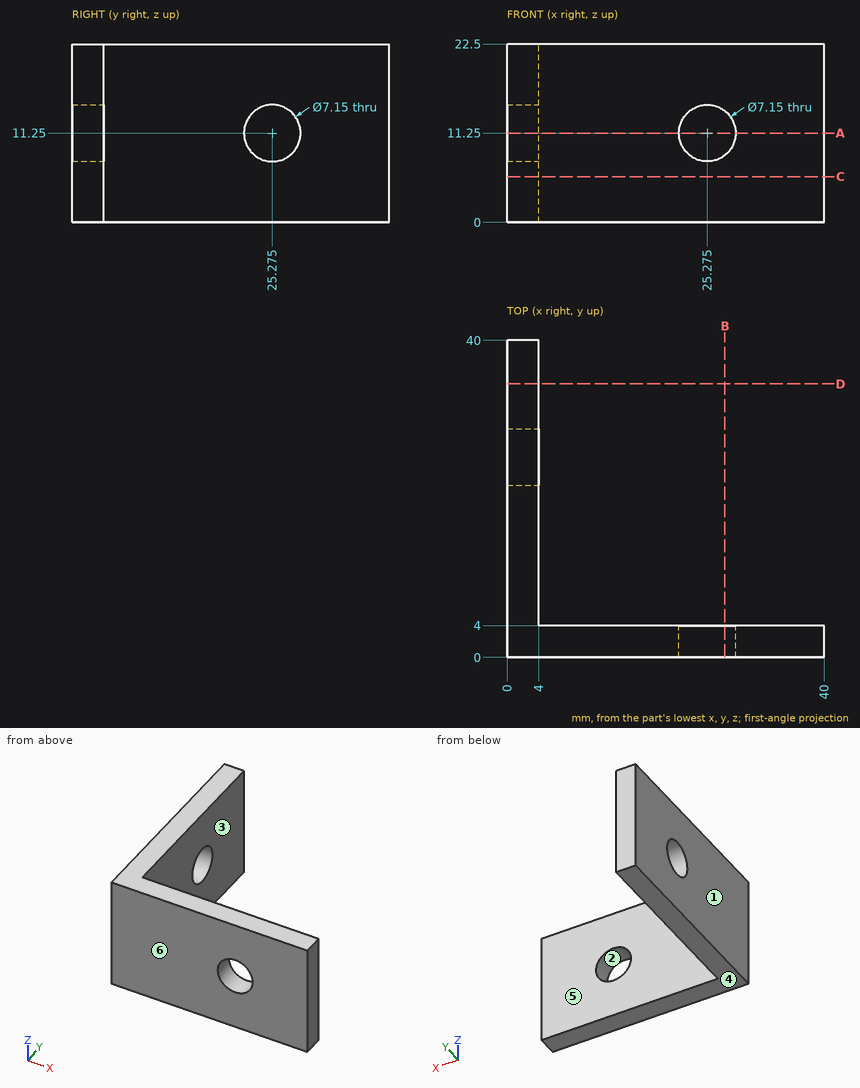
Could you check a few things on this drawing? It's one solid part, dimensions in mm from its lowest x, y, z. A direction names the side the tool comes from. Give positions to 0.01 mm unless a question says otherwise; leave off trailing zeros. Order: outer loops, then holes, each group sorted by start corner. A loop starts at its lowest first (then second) coordinate and runs counter-clockwise, first axis right, second up.
1. Which directions (+Z, -Z, +X, -X, +Y, -Y) give clear straight access to the entire face, cutting with the end or side of a thin tool? Please do the marked faces 5 and 6.
Answers below:
face 5: +Z, -Z, +X, +Y
face 6: +Z, -Z, +X, -X, -Y
2. Suppose I cut it at D-D (y = 34.5). Write out the boundary of the cut face in (x, z).
Answers below:
outline: (0, 0) - (4, 0) - (4, 22.5) - (0, 22.5) - close
3. I need wall thicknesses on L1, parallel to X at y = 3.2, z = 11.25; L2, parallel to Y at x = 5, z = 19.25. Which ranges of each line are inside material? Lowest first, please.
Answers below:
L1: x = 0 to 21.7, 28.85 to 40
L2: y = 0 to 4
4. Suppose I cut it at C-C (z = 5.75). Write out the boundary of the cut face in (x, y), plus the area to 3 significant figures.
Answers below:
outline: (0, 0) - (40, 0) - (40, 4) - (4, 4) - (4, 40) - (0, 40) - close
area: 304 mm2
5. Thinking about a two-plate mould opening in X: for the marked faces 1, 2, 3 and 4, which applies, +X half, -X half, draft (parallel to the pull), parting line (faces both ways), or undercut?
Answers below:
face 1: -X half
face 2: undercut
face 3: +X half
face 4: draft
6. Suppose I cut it at A-A (z = 11.25). Write out the boundary of the cut face in (x, y), plus the area to 3 significant figures.
Answers below:
outline: (0, 0) - (21.7, 0) - (21.7, 4) - (4, 4) - (4, 21.7) - (0, 21.7) - close; (0, 28.85) - (4, 28.85) - (4, 40) - (0, 40) - close; (28.85, 0) - (40, 0) - (40, 4) - (28.85, 4) - close
area: 247 mm2
7. Suppose I cut it at B-B (x = 27.5). Write out the boundary of the cut face in (y, z).
Answers below:
outline: (0, 0) - (4, 0) - (4, 8.45) - (0, 8.45) - close; (0, 14.05) - (4, 14.05) - (4, 22.5) - (0, 22.5) - close
8. For pin 1 (11 mm diameter, centred on y = 27, z = 8, fed in from +X), with a flat end and sliding along its axis, tell me the tip position at first contact or that it passes through.
Answers below:
pin 1: stops at x = 4
